Model file for the job. Use its own axes, mm. A direction names the side the tool comes from. Coordinates: 2 decimals unless noted, no trailing zeros. Loops run counter-clockwise (first coordinate to the right, second up) from the corner with the lowest first, then second, coordinate; pieces in that order, holes last. Notation, with made-up numbers: (71.5, -6.5) -> (84.5, -6.5) arc R36 cw to (84.5, 31.5) -> close; hole circle Ø9 at (74, 83.5). An arc over 180 degrees is marked (long way). Use one line per item in the form item = value.
```python
from build123d import *

# Parameters (mm, degrees)
SKETCH1_R           = 90
SKETCH1_R_2         = 61
BOSS_EXTRUDE1_DEPTH = 35
SKETCH2_R           = 59
CUT_EXTRUDE1_DEPTH  = 71
CIRPATTERN1_COUNT   = 20
CUT_EXTRUDE2_START  = -35
SKETCH3_R           = 90
SKETCH3_R_2         = 80
CUT_EXTRUDE2_DEPTH  = 12.5


with BuildPart() as part:
    # Sketch1 → Boss-Extrude1 (new body, symmetric)
    with BuildSketch(Plane(origin=(0, 0, 0), x_dir=(0, 0, -1), z_dir=(1, 0, 0))):
        Circle(SKETCH1_R)
        Circle(SKETCH1_R_2, mode=Mode.SUBTRACT)
    extrude(amount=BOSS_EXTRUDE1_DEPTH, both=True)

    # Sketch2 → Cut-Extrude1 (cut, through all)
    with BuildSketch(Plane(origin=(35, 0, 0), x_dir=(0, 0, -1), z_dir=(1, 0, 0))):
        Circle(SKETCH2_R)
        with BuildLine():
            Line((0, 51.395835648), (-4.5, 58.828139525))
            Line((-4.5, 58.828139525), (-5.415254237, 70.793184852))
            ThreePointArc((-5.415254237, 70.793184852), (0.535268123, 70.997982281), (6.48202623, 70.703488853))
            Line((6.48202623, 70.703488853), (4.5, 58.828139525))
            Line((4.5, 58.828139525), (0, 51.395835648))
        make_face()
    cut_extrude1 = extrude(amount=-CUT_EXTRUDE1_DEPTH, mode=Mode.SUBTRACT)

    # CirPattern1: Cut-Extrude1 ×20 about axis
    cirpattern1_axis = Axis((0, 0, 0), (1, 0, 0))
    for i in range(1, CIRPATTERN1_COUNT):
        add(cut_extrude1.rotate(cirpattern1_axis, i * 360 / CIRPATTERN1_COUNT), mode=Mode.SUBTRACT)

    # Sketch3 → Cut-Extrude2 (cut, symmetric)
    with BuildSketch(Plane(origin=(35, 0, 0), x_dir=(0, 0, -1), z_dir=(1, 0, 0)).offset(CUT_EXTRUDE2_START)):
        Circle(SKETCH3_R)
        Circle(SKETCH3_R_2, mode=Mode.SUBTRACT)
    extrude(amount=CUT_EXTRUDE2_DEPTH, both=True, mode=Mode.SUBTRACT)


solid = part.part
```
Q1. Band-saw the part on C-C, the plane z = 43. Write the cut outline in (x, y).
Result:
outline = (-35, -79.06) -> (-12.5, -79.06) -> (-12.5, -67.46) -> (12.5, -67.46) -> (12.5, -79.06) -> (35, -79.06) -> (35, -56.5) -> (-35, -56.5) -> close; (-35, -49.65) -> (35, -49.65) -> (35, -43.27) -> (-35, -43.27) -> close; (-35, 43.27) -> (35, 43.27) -> (35, 50.57) -> (-35, 50.57) -> close; (-35, 56.5) -> (35, 56.5) -> (35, 79.06) -> (12.5, 79.06) -> (12.5, 67.46) -> (-12.5, 67.46) -> (-12.5, 79.06) -> (-35, 79.06) -> close
Q2. Pin check, flat tips, straight feed: pin 1 Ø12 at (x, z) = (14.5, -35) entering from +Y; pin 2 Ø4 at (x, z) = (4.5, 56) entering from +Y; pin 3 Ø5 at (x, y) = (24, 18.5) entering from -Z. Stop position of each tip, or through.
Result:
pin_1 = 85.2
pin_2 = 59.03
pin_3 = -88.57
Q3. Which spindle directions (+Z, -Z, +X, -X, +Y, -Y) get a long thin tool onto all of the face, cutting with end or side? Do faces 1 (the face through (0.49, 50.23, 42.71)), 2 (the face through (-35, 60, -13)). Say none if no direction does.
Result:
face_1 = +X, -X
face_2 = +Z, -Z, -X, +Y, -Y
Q4. Wall check: line 1 along X through (y, z) = (-28.5, 82); line 2 along Z through (x, y) = (-15, -58); line 3 along Z through (x, y) = (-7, 1.5). Give the ranges that are in metal, low to high.
Result:
line_1 = -35 to -12.5, 12.5 to 35
line_2 = -68.82 to -40.95, -34.81 to -23.88, 24.25 to 35.72, 40.95 to 68.82
line_3 = -79.99 to -70.98, 70.98 to 79.99
Q5. Band-saw the part on A-A, the plane y = 0. Write the cut outline in (x, z).
Result:
outline = (-35, -90) -> (-12.5, -90) -> (-12.5, -80) -> (12.5, -80) -> (12.5, -90) -> (35, -90) -> (35, -71) -> (-35, -71) -> close; (-35, 71) -> (35, 71) -> (35, 90) -> (12.5, 90) -> (12.5, 80) -> (-12.5, 80) -> (-12.5, 90) -> (-35, 90) -> close
